Autodesk Inventor part; units mm, degrees
ref_plane "YZ Plane" through (0, 0, 0) normal (1, 0, 0) x (0, 1, 0)
ref_plane "XZ Plane" through (0, 0, 0) normal (0, 1, 0) x (-1, 0, 0)
ref_plane "XY Plane" through (0, 0, 0) normal (0, 0, 1) x (1, 0, 0)
sketch "Sketch1" plane through (0, 0, 0) normal (0, 0, 1) x (1, 0, 0)
  circle A0 centre (0, 0) radius 19
  dimension "d0" = 38
extrude "Extrusion1" add sketch "Sketch1" along normal blind 57.1
sketch "Sketch2" plane through (0, 0, 57.1) normal (0, 0, 1) x (1, 0, 0)
  circle A0 centre (0, 0) radius 16
  dimension "d3" = 32
extrude "Extrusion2" add sketch "Sketch2" along normal blind 41.8
sketch "Sketch3" plane through (0, 0, 98.9) normal (0, 0, 1) x (1, 0, 0)
  circle A0 centre (0, 0) radius 10
  dimension "d6" = 20
extrude "Extrusion3" add sketch "Sketch3" along normal blind 3
sketch "Sketch4" plane through (0, 0, 101.9) normal (0, 0, 1) x (1, 0, 0)
  circle A0 centre (0, 0) radius 3
  dimension "d9" = 6
extrude "Extrusion4" add sketch "Sketch4" along normal blind 16.2
sketch "Sketch5" plane through (0, 0, 101.9) normal (0, 0, 1) x (1, 0, 0)
  line L0 (-9, -9) -> (9, -9) construction
  line L1 (9, -9) -> (9, 9) construction
  line L2 (9, 9) -> (-9, 9) construction
  line L3 (-9, 9) -> (-9, -9) construction
  line L4 (-9, -9) -> (9, 9) construction
  line L5 (9, -9) -> (-9, 9) construction
  circle A0 centre (9, 9) radius 1.5
  circle A1 centre (9, -9) radius 1.5
  circle A2 centre (-9, -9) radius 1.5
  circle A3 centre (-9, 9) radius 1.5
  point P0 (0, 0)
  dimension "d12" = 18
  dimension "d13" = 18
  dimension "d14" = 3
  dimension "d15" = 3
  dimension "d16" = 3
  dimension "d17" = 3
extrude "Extrusion5" cut sketch "Sketch5" against normal blind 25
sketch "Sketch6" plane through (0, 0, 98.9) normal (0, 0, 1) x (1, 0, 0)
  circle A0 centre (0, 0) radius 3
  circle A1 centre (0, 0) radius 10
  line L0 (-4.3589, -9) -> (4.3589, -9)
  line L1 (-4.3589, 9) -> (4.3589, 9)
  dimension "d20" = 18
extrude "Extrusion6" cut sketch "Sketch6" along normal through all contours L1 A1 | A1 L0
properties part number "12RPM Gear Motor"
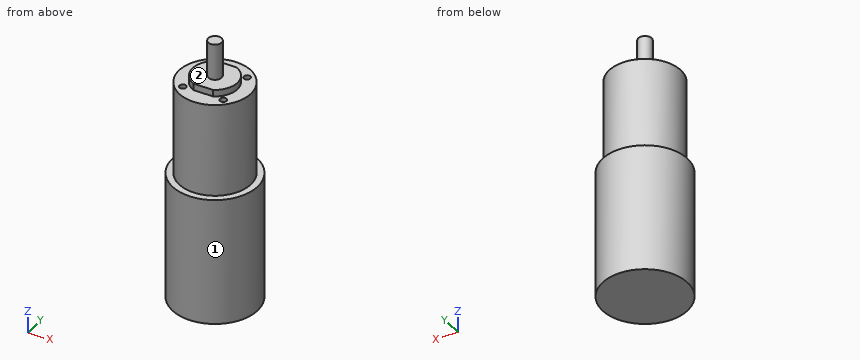
CAD build for the part. Positions are in the model's coordinates, mm. Face numbers are marked on the shaded views. A direction names the side the tool comes from. Round coordinates to 2 decimals unless told otherwise and drop trailing zeros. Write each loop counter-clockwise with the first axis right and the second up, starting at its lowest first coordinate (ties: lowest second). Pieces come first, ordered by that corner, then holes. Notation, with made-up numbers: (-0.75, 20.25) - (34.25, 20.25) arc R23 ccw to (34.25, 56.25) - close; hole circle Ø11 at (31, 23.5). An arc over 180 degrees is marked (long way). Write item = value, one per line. Start each with the question number.
Q1. Which spindle directions (+Z, -Z, +X, -X, +Y, -Y) get a long thin tool onto all of the face, cutting with end or side? Do the marked faces 1 and 2. Say none if no direction does.
Q2. Band-saw the part on B-B (x = 0). Give the cut face in (y, z).
Q3. Probe L1, parallel to Y at x = -9, z = 92.25; L2, parallel to Z at x = -4, y = 6.5; L3, parallel to X at y = 8.5, z = 98. List the from-to ranges inside material, lowest first. Write a range as from..to.
Q4. Band-saw the part on C-C (y = 4.5). Give the cut face in (x, z).
Q5. Band-saw the part on A-A (z = 96.5). Give the cut face in (x, y).
Q6. Band-saw the part on D-D (z = 52.5). Give the cut face in (x, y), then the cut area to 3 significant figures.
Q7. Drop flat-ended pins along their axis: pin 1 (1 mm diameter, centred on y = -14.5, z = 91, fed in from -X); pin 2 (1.8 mm diameter, centred on x = -9, y = 9, fed in from +Z); pin 3 (2.5 mm diameter, centred on x = 2, z = 100.5, fed in from +Y). Give the stop position or say it passes through.
Answers below:
q1.face_1 = +Z, -Z
q1.face_2 = +Z
q2.outline = (-19, 0) - (19, 0) - (19, 57.1) - (16, 57.1) - (16, 98.9) - (9, 98.9) - (9, 101.9) - (3, 101.9) - (3, 118.1) - (-3, 118.1) - (-3, 101.9) - (-9, 101.9) - (-9, 98.9) - (-16, 98.9) - (-16, 57.1) - (-19, 57.1) - close
q3.L1 = -13.23..-10.5, -7.5..7.5, 10.5..13.23
q3.L2 = 0..101.9
q3.L3 = -13.56..-10.41, -7.59..7.59, 10.41..13.56
q4.outline = (-18.46, 0) - (18.46, 0) - (18.46, 57.1) - (15.35, 57.1) - (15.35, 98.9) - (8.93, 98.9) - (8.93, 101.9) - (-8.93, 101.9) - (-8.93, 98.9) - (-15.35, 98.9) - (-15.35, 57.1) - (-18.46, 57.1) - close
q5.outline = circle Ø32 at (0, 0); hole circle Ø3 at (-9, -9); hole circle Ø3 at (-9, 9); hole circle Ø3 at (9, -9); hole circle Ø3 at (9, 9)
q6.outline = circle Ø38 at (0, 0)
q6.area = 1,130 mm2
q7.pin_1 = -7.75
q7.pin_2 = 76.9
q7.pin_3 = 9
